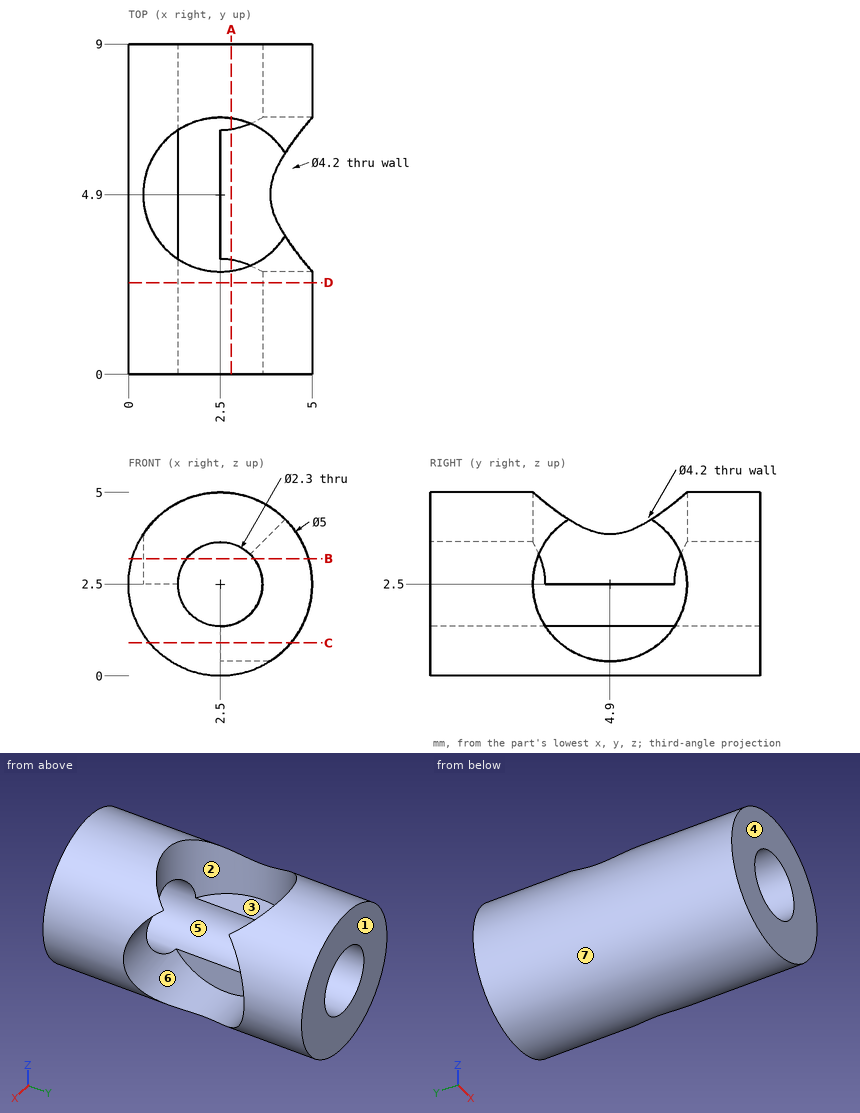
Part print with two shaded views. Sizes in mm from the minimum x, y, z corner. A direction names the side the tool comes from. Round coordinates to 2 decimals unless told otherwise and drop trailing zeros. Order: outer loops, then holes, each group sorted by start corner. A loop starts at its lowest first (then second) coordinate and runs counter-clockwise, first axis right, second up. Notation, with made-up numbers: M 31.25,-33 L 64.25,-33 A35 cw 64.25,0 Z; hole C -7,72.5 d8. An arc over 180 degrees is marked long. Put each result on its own line as item: value. Start each with the question number.
1. Slice it at B-B on z = 3.2. List the corners of the cut face in (x, y).
2. Slice it at A-A on x = 2.8. List the corners of the cut face in (y, z).
3. Drop flat-ended pins along their axis: pin 1 (0.8 mm diameter, centred on x = 0.5, y = 5, fed in from +Z) (3 decimals); pin 2 (1.8 mm diameter, centred on x = 2.5, z = 2.5, fed in from -Y). Give the stop position or say it passes through.
4. Slice it at D-D on y = 2.5. List the corners of the cut face in (x, z), then the cut area to 3 significant figures.
5. Tool access for the marked faces 1, 2 and 3: list every direction of +Z, -Z, +X, -X, +Y, -Y with a clear straight run to the whole face (end or side of a thin tool).
6. Slice it at C-C on z = 0.9. List the corners of the cut face in (x, y), then the cut area to 3 significant figures.
7. Drill centre lines: probe 1 along X at (y, z) = (1.5, 1.6); probe 2 along Z at (x, y) = (1.5, 7.25); probe 3 along Y at (x, z) = (4.1, 1.3). Where is each one in solid material? Low to high. Write a range as [from, to].
8. Two-plate mould, pull along Z, no slides. Class the marked faces 4, 5, 6 and 7: +Z half, -Z half, draft (parallel to the pull), parting line (faces both ways), or undercut.
Findings:
1. outline: M 0.1,0 L 1.59,0 L 1.59,3.01 A2.1 cw 1.59,6.79 L 1.59,9 L 0.1,9 Z; M 3.41,0 L 4.9,0 L 4.9,2.92 L 3.41,2.92 Z; M 3.41,6.88 L 4.9,6.88 L 4.9,9 L 3.41,9 Z
2. outline: M 0,0.02 L 9,0.02 L 9,1.39 L 6.68,1.39 A2.1 cw 3.12,1.39 L 0,1.39 Z; M 0,3.61 L 2.82,3.61 L 2.82,4.98 L 0,4.98 Z; M 6.98,3.61 L 9,3.61 L 9,4.98 L 6.98,4.98 Z
3. pin 1: z = 3.945
3. pin 2: through
4. outline: C 2.5,2.5 d5; hole C 2.5,2.5 d2.3
4. area: 15.5 mm2
5. face 1: +Z, -Z, +X, -X, +Y
5. face 2: +Z
5. face 3: +Z, +X
6. outline: M 0.58,0 L 4.42,0 L 4.42,3.54 L 2.5,3.54 L 2.5,6.26 L 4.42,6.26 L 4.42,9 L 0.58,9 Z
6. area: 29.4 mm2
7. probe 1: [0.17, 1.78], [3.22, 4.83]
7. probe 2: [0.21, 1.93], [3.07, 4.79]
7. probe 3: [0, 3.18], [6.62, 9]
8. face 4: draft
8. face 5: undercut
8. face 6: undercut
8. face 7: parting line
